Here's how the part is built. I have some questions about the finished solid (model axes, mm). A direction names the side the tool comes from. Coordinates: 2 decimals unless noted, no trailing zeros. Write each loop counter-clockwise with the first axis right and the second up, starting at its lowest first coordinate (ties: lowest second). Pieces come first, ordered by that corner, then holes.
from build123d import *

# Parameters (mm, degrees)
F0_R        = 10.16
F1_DEPTH    = 5.08
F2_R        = 12.7
F2_R_2      = 10.16
F3_DEPTH    = 5.08
F5_DEPTH    = 25.4
F6_T1_DEPTH = 88.4028561312
F7_W        = 6.1679999344
F7_H        = 12.5403126109
F8_DEPTH    = 5.08


# Not quite as in the source:
# - a fillet or chamfer that OpenCascade refuses, or shapes differently, is made with other operations: its cross-section is extruded or revolved along the edge and cut away or added


with BuildPart() as f1:
    # F0 (on Top) → F1 (new body)
    with BuildSketch(Plane.XY):
        Circle(F0_R)
    extrude(amount=F1_DEPTH)

    # F2 (on face) → F3 (join)
    with BuildSketch(Plane.XY.offset(5.08)):
        Circle(F2_R)
        Circle(F2_R_2, mode=Mode.SUBTRACT)
        Circle(F2_R_2)
    extrude(amount=F3_DEPTH)

    # F4 (on face) → F5 (join)
    with BuildSketch(Plane.XY.offset(10.16)):
        with BuildLine():
            Line((-5.3003839328, -11.5410541184), (0, -11.5410541184))
            Line((0, -11.5410541184), (5.3003839328, -11.5410541184))
            ThreePointArc((5.3003839328, -11.5410541184), (7.254211996, -10.4243181224), (8.9802561211, -8.9802561211))
            ThreePointArc((8.9802561211, -8.9802561211), (10.4243181224, -7.254211996), (11.5410541184, -5.3003839328))
            Line((11.5410541184, -5.3003839328), (11.5410541184, 0))
            Line((11.5410541184, 0), (11.5410541184, 5.3003839328))
            ThreePointArc((11.5410541184, 5.3003839328), (8.9802561211, 8.9802561211), (5.3003839328, 11.5410541184))
            Line((5.3003839328, 11.5410541184), (-5.3003839328, 11.5410541184))
            ThreePointArc((-5.3003839328, 11.5410541184), (-8.9802561211, 8.9802561211), (-11.5410541184, 5.3003839328))
            Line((-11.5410541184, 5.3003839328), (-11.5410541184, -5.3003839328))
            ThreePointArc((-11.5410541184, -5.3003839328), (-8.9802561211, -8.9802561211), (-5.3003839328, -11.5410541184))
        make_face()
        with BuildLine():
            Line((-11.5410541184, -11.5410541184), (-5.3003839328, -11.5410541184))
            ThreePointArc((-5.3003839328, -11.5410541184), (-8.9802561211, -8.9802561211), (-11.5410541184, -5.3003839328))
            Line((-11.5410541184, -5.3003839328), (-11.5410541184, -11.5410541184))
        make_face()
        with BuildLine():
            Line((8.9802561211, -8.9802561211), (11.5410541184, -11.5410541184))
            Line((11.5410541184, -11.5410541184), (11.5410541184, -5.3003839328))
            ThreePointArc((11.5410541184, -5.3003839328), (10.4243181224, -7.254211996), (8.9802561211, -8.9802561211))
        make_face()
        with BuildLine():
            ThreePointArc((8.9802561211, -8.9802561211), (7.254211996, -10.4243181224), (5.3003839328, -11.5410541184))
            Line((5.3003839328, -11.5410541184), (11.5410541184, -11.5410541184))
            Line((11.5410541184, -11.5410541184), (8.9802561211, -8.9802561211))
        make_face()
        with BuildLine():
            Line((-11.5410541184, 11.5410541184), (-11.5410541184, 5.3003839328))
            ThreePointArc((-11.5410541184, 5.3003839328), (-8.9802561211, 8.9802561211), (-5.3003839328, 11.5410541184))
            Line((-5.3003839328, 11.5410541184), (-11.5410541184, 11.5410541184))
        make_face()
        with BuildLine():
            ThreePointArc((5.3003839328, 11.5410541184), (8.9802561211, 8.9802561211), (11.5410541184, 5.3003839328))
            Line((11.5410541184, 5.3003839328), (11.5410541184, 11.5410541184))
            Line((11.5410541184, 11.5410541184), (5.3003839328, 11.5410541184))
        make_face()
    extrude(amount=F5_DEPTH)

    # F6: chamfer of 12.7 on 2 edges, made by hand

    # F6_s2 → F6_t1 (cut)
    with BuildSketch(Plane.XZ.offset(-44.2014280656)):
        Polygon((11.5410541184, 22.86), (-1.1589458816, 35.56), (11.5410541184, 35.56), align=None)
        Polygon((-11.5410541184, 22.86), (1.1589458816, 35.56), (-11.5410541184, 35.56), align=None)
    extrude(amount=F6_T1_DEPTH, mode=Mode.SUBTRACT)

    # F7 (on face) → F8 (cut)
    with BuildSketch(Plane.XZ.offset(11.5410541184)):
        with Locations((0, 16.4301563054)):
            Rectangle(F7_W, F7_H)
    extrude(amount=-F8_DEPTH, mode=Mode.SUBTRACT)


solid = f1.part
1. I want a section at C-C (z = 21). List the corners of the cut face in (x, y) for me.
2. If I drill on line 1 (X direction, y = -8.25, z = 11); line 2 (X direction, y = 6, z = 14); line 3 (Y direction, x = -2.5, z = 15), over which ranges is the centre line in solid material (lowest first)?
3. I want a section at D-D (y = 5.75). List the corners of the cut face in (x, z) for me.
4. For pin 1 Ø1.9 at (x, y) = (8.5, 7.5) entering from -Z; pin 2 Ø1.3 at (x, y) = (-1.5, 12) entering from +Z; pin 3 Ø10 at (y, z) = (5, 19.5) entering from -X, each with a flat end and sliding along its axis, tell me the tip position at first contact or that it passes through.
5. On a 3-axis mill with a long thin cutter (end or side, diameter ignored), from which of +Z, -Z, +X, -X, +Y, -Y can I reach the whole of each face in a straight line? I mean faces 1 (the face through (-2.75, -12.4, 7.58)), 2 (the face through (-3.084, -9, 16)), 3 (the face through (12, 0, 10.16)). Say none if no direction works.
6. I want a section at B-B (x = 0.75). List the corners of the cut face in (y, z) for me.
7. I want a section at A-A (y = 0). List the corners of the cut face in (x, z) for me, then the cut area to 3 significant figures.
8. Thinking about a two-plate mould opening in X: for faces 4 (the face through (-5.9, 0.2, 28.5)), 5 (the face through (0, -9, 22.7)), 6 (the face through (3.084, -9, 16)), 7 (the face through (10, -10, 10.16)), which applies, pulls with the +X half, pulls with the -X half, needs draft (parallel to the pull), parting line crosses it, or undercut?
Response values:
1. outline: (-11.54, -11.54) - (-3.08, -11.54) - (-3.08, -6.46) - (3.08, -6.46) - (3.08, -11.54) - (11.54, -11.54) - (11.54, 11.54) - (-11.54, 11.54) - close
2. line 1: x = -11.54 to -3.08, 3.08 to 11.54
2. line 2: x = -11.54 to 11.54
2. line 3: y = -6.46 to 11.54
3. outline: (-11.54, 10.16) - (-11.32, 10.16) - (-11.32, 5.08) - (-8.38, 5.08) - (-8.38, 0) - (8.38, 0) - (8.38, 5.08) - (11.32, 5.08) - (11.32, 10.16) - (11.54, 10.16) - (11.54, 22.86) - (0, 34.4) - (-11.54, 22.86) - close
4. pin 1: stops at z = 5.08
4. pin 2: stops at z = 33.36
4. pin 3: stops at x = -11.54
5. face 1: -Z
5. face 2: -Y
5. face 3: +Z, +X, +Y, -Y
6. outline: (-12.68, 5.08) - (-10.13, 5.08) - (-10.13, 0) - (10.13, 0) - (10.13, 5.08) - (12.68, 5.08) - (12.68, 10.16) - (11.54, 10.16) - (11.54, 33.65) - (-11.54, 33.65) - (-11.54, 22.7) - (-6.46, 22.7) - (-6.46, 10.16) - (-12.68, 10.16) - close
7. outline: (-12.7, 5.08) - (-10.16, 5.08) - (-10.16, 0) - (10.16, 0) - (10.16, 5.08) - (12.7, 5.08) - (12.7, 10.16) - (11.54, 10.16) - (11.54, 22.86) - (0, 34.4) - (-11.54, 22.86) - (-11.54, 10.16) - (-12.7, 10.16) - close
7. area: 659 mm2
8. face 4: pulls with the -X half
8. face 5: undercut
8. face 6: undercut
8. face 7: needs draft
